Could you check a few things on this model? Use its own coordinates, in mm. Face numbers are marked on the shaded views. Round coordinates to 2 decimals unless told otherwise and drop trailing zeros. Order: outer loops, then holes, each group sorted by start corner. A loop starts at its lowest first (then second) coordinate and runs counter-clockwise, first axis right, second up. Notation, with made-up numbers: (35, -21) - (85, -21) arc R11 cw to (85, -8) - close; hole circle Ø4 at (56, 73). An arc over 180 degrees is marked (long way). Use one line per item in the form item = value.
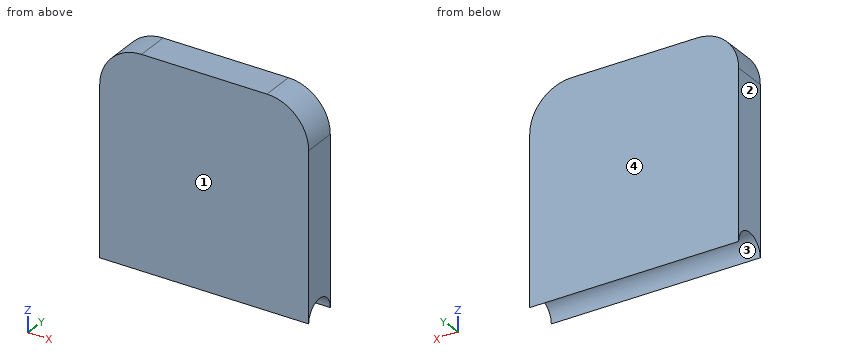
from build123d import *

# Parameters (mm, degrees)
F0_W     = 25
F0_H     = 25
F1_DEPTH = 4
F2_R     = 5
F4_D     = 4


with BuildPart() as f1:
    # F0 (on Front) → F1 (new body)
    with BuildSketch(Plane.XZ):
        with Locations((0, 12.5)):
            Rectangle(F0_W, F0_H)
    extrude(amount=F1_DEPTH)

    # F2
    f2_edges = [f1.edges().sort_by_distance(p)[0] for p in [
        (-12.5, -2, 25),
        (12.5, -2, 25),
    ]]
    fillet(f2_edges, radius=F2_R)

    # F4 (through all)
    with Locations(Plane.YZ.offset(12.5)):
        with Locations((-2, 0)):
            Hole(F4_D / 2)


solid = f1.part
Item 1: Will these pins go through, and if not, where does the flat tip stop? P1, Ø1.5, axis at x = 9, y = -1, coming from the +Z side; P2, Ø1, axis at x = -1, y = -3, coming from the -Z side; P3, Ø1, axis at x = -6, z = 19.5, coming from the +Y side.
Found:
P1 = 24.94
P2 = 1.32
P3 = 0
Item 2: If we mould it in two halves opening along Y, with no side actions, what happens to the marked faces 1, 2, 3 and 4? For each: released by +Y, released by -Y, zero draft, split by the parting line, or undercut.
Found:
face_1 = released by -Y
face_2 = zero draft
face_3 = undercut
face_4 = released by +Y
Item 3: Imagine slicing it at B-B on x = 3.75. Please give me the cut outline in (y, z), plus the area to 3 significant figures.
Found:
outline = (-4, 0) arc R2 cw to (0, 0) - (0, 25) - (-4, 25) - close
area = 93.7 mm2
Item 4: Imagine slicing it at A-A on y = -2. Please give me the cut outline in (x, z), plus the area to 3 significant figures.
Found:
outline = (-12.5, 2) - (12.5, 2) - (12.5, 20) arc R5 ccw to (7.5, 25) - (-7.5, 25) arc R5 ccw to (-12.5, 20) - close
area = 564 mm2
Item 5: I need wall thicknesses on L1, parallel to X at y = -1.15, z = 20.5; L2, parallel to Z at x = -4.5, y = -0.6; L3, parallel to Z at x = 8.25, y = -3.45. Which ranges of each line are inside material? Lowest first, please.
Found:
L1 = -12.47 to 12.47
L2 = 1.43 to 25
L3 = 1.38 to 24.94
Item 6: Imagine slicing it at C-C on y = -0.6. Please give me the cut outline in (x, z), plus the area to 3 significant figures.
Found:
outline = (-12.5, 1.43) - (12.5, 1.43) - (12.5, 20) arc R5 ccw to (7.5, 25) - (-7.5, 25) arc R5 ccw to (-12.5, 20) - close
area = 579 mm2
Item 7: Imagine slicing it at D-D on x = 8. Please give me the cut outline in (y, z).
Found:
outline = (-4, 0) arc R2 cw to (0, 0) - (0, 24.97) - (-4, 24.97) - close
